Can you work these out from the model? Positions are in its coordinate system, mm. A direction names the side the tool comes from. Give positions to 0.01 mm unless a question says otherwise; leave off trailing zeros. Loops run counter-clockwise (first coordinate to the right, second up) from the corner with the lowest first, then second, coordinate; pieces in that order, holes last. Notation, with made-up numbers: (20.25, 67) -> (44.25, 67) arc R31 cw to (44.25, 101) -> close; hole circle Ø10 at (82, 59.5). An arc over 180 degrees is marked (long way). Use CSV: the item, a comma, the result in double quotes.
from build123d import *

# Parameters (mm, degrees)
SKETCH1_W           = 60
SKETCH1_H           = 60
BOSS_EXTRUDE1_DEPTH = 6
CUT_EXTRUDE2_DEPTH  = 3
SKETCH12_R          = 1.15
CUT_EXTRUDE9_DEPTH  = 43.848570571
SKETCH5_W           = 20
SKETCH5_H           = 60
BOSS_EXTRUDE2_DEPTH = 7
SKETCH6_R           = 1.15
CUT_EXTRUDE4_DEPTH  = 45.373415465
SKETCH8_R           = 2.2
SKETCH8_R_2         = 1.15
CUT_EXTRUDE5_DEPTH  = 9
CUT_EXTRUDE6_DEPTH  = 10
SKETCH10_W          = 6
SKETCH10_H          = 33.5
CUT_EXTRUDE7_DEPTH  = 3
CUT_EXTRUDE8_DEPTH  = 66.711490624


with BuildPart() as part:
    # Sketch1 → Boss-Extrude1 (new body)
    with BuildSketch(Plane.XY):
        Rectangle(SKETCH1_W, SKETCH1_H)
    extrude(amount=BOSS_EXTRUDE1_DEPTH)

    # Sketch3 → Cut-Extrude2 (cut)
    with BuildSketch(Plane(origin=(0, 0, 0), x_dir=(-1, 0, 0), z_dir=(0, 0, -1))):
        Polygon((2.1, 6.287564435), (2.1, 8.712435565), (0, 9.924871131), (-2.1, 8.712435565), (-2.1, 6.287564435), (0, 5.075128869), align=None)
        Polygon((2.1, -8.712435565), (2.1, -6.287564435), (0, -5.075128869), (-2.1, -6.287564435), (-2.1, -8.712435565), (0, -9.924871131), align=None)
        Polygon((2.1, -23.712435565), (2.1, -21.287564435), (0, -20.075128869), (-2.1, -21.287564435), (-2.1, -23.712435565), (0, -24.924871131), align=None)
        Polygon((0, 20.075128869), (2.1, 21.287564435), (2.1, 23.712435565), (0, 24.924871131), (-2.1, 23.712435565), (-2.1, 21.287564435), align=None)
    extrude(amount=-CUT_EXTRUDE2_DEPTH, mode=Mode.SUBTRACT)

    # Sketch12 → Cut-Extrude9 (cut, through all)
    with BuildSketch(Plane(origin=(0, 0, 0), x_dir=(-1, 0, 0), z_dir=(0, 0, -1))):
        with Locations((0, 22.5)):
            Circle(SKETCH12_R)
        with Locations((0, 7.5)):
            Circle(SKETCH12_R)
        with Locations((0, -7.5)):
            Circle(SKETCH12_R)
        with Locations((0, -22.5)):
            Circle(SKETCH12_R)
    extrude(amount=-CUT_EXTRUDE9_DEPTH, mode=Mode.SUBTRACT)

    # Sketch5 → Boss-Extrude2 (add)
    with BuildSketch(Plane.XY.offset(6)):
        with Locations((-20, 0)):
            Rectangle(SKETCH5_W, SKETCH5_H)
        with Locations((20, 0)):
            Rectangle(SKETCH5_W, SKETCH5_H)
    extrude(amount=BOSS_EXTRUDE2_DEPTH)

    # Sketch6 → Cut-Extrude4 (cut, through all)
    with BuildSketch(Plane.XY.offset(13)):
        with Locations((-25, 25)):
            Circle(SKETCH6_R)
        with Locations((25, 25)):
            Circle(SKETCH6_R)
        with Locations((25, -25)):
            Circle(SKETCH6_R)
        with Locations((-25, -25)):
            Circle(SKETCH6_R)
    extrude(amount=-CUT_EXTRUDE4_DEPTH, mode=Mode.SUBTRACT)

    # Sketch8 → Cut-Extrude5 (cut)
    # profile 1 of 4: a face of its own
    with BuildSketch(Plane.XY.offset(13)):
        with Locations((-25, 25)):
            Circle(SKETCH8_R)
        with Locations((-25, 25)):
            Circle(SKETCH8_R_2, mode=Mode.SUBTRACT)
    # profile 2 of 4: a face of its own
    with BuildSketch(Plane.XY.offset(13)):
        with Locations((25, 25)):
            Circle(SKETCH8_R)
    # profile 3 of 4: a face of its own
    with BuildSketch(Plane.XY.offset(13)):
        with Locations((25, -25)):
            Circle(SKETCH8_R)
    # profile 4 of 4: a face of its own
    with BuildSketch(Plane.XY.offset(13)):
        with Locations((-25, -25)):
            Circle(SKETCH8_R)
        with Locations((-25, -25)):
            Circle(SKETCH8_R_2, mode=Mode.SUBTRACT)
    extrude(amount=-CUT_EXTRUDE5_DEPTH, mode=Mode.SUBTRACT)

    # Sketch9 → Cut-Extrude6 (cut)
    with BuildSketch(Plane.XY.offset(13)):
        Polygon((-25, -16.55), (-15.5, -27), (-10, -27), (-10, 6.5), (-23.375, 6.5), (-25, 4.9), (-25, 3.3), (-27, 3.3), (-27, -3.3), (-25, -3.3), align=None)
    extrude(amount=-CUT_EXTRUDE6_DEPTH, mode=Mode.SUBTRACT)

    # Sketch10 → Cut-Extrude7 (cut)
    with BuildSketch(Plane.XY.offset(6)):
        with Locations((-7, -10.25)):
            Rectangle(SKETCH10_W, SKETCH10_H)
    extrude(amount=-CUT_EXTRUDE7_DEPTH, mode=Mode.SUBTRACT)

    # Sketch11 → Cut-Extrude8 (cut, through all)
    with BuildSketch(Plane(origin=(-27, 0, 0), x_dir=(0, 0, -1), z_dir=(1, 0, 0))):
        with BuildLine():
            Line((-3, -0.899652711), (-3, 0.899652711))
            ThreePointArc((-3, 0.899652711), (-9.475, 0), (-3, -0.899652711))
        make_face()
    extrude(amount=-CUT_EXTRUDE8_DEPTH, mode=Mode.SUBTRACT)


solid = part.part
(1) If we section it at B-B, the plane z = 7.5: Write out the boundary of the cut face in (x, y) (3 decimals), then the cut area to 3 significant figures.
Answer sheet:
outline,"(-30, -30) -> (-10, -30) -> (-10, -27) -> (-15.5, -27) -> (-25, -16.55) -> (-25, -3.3) -> (-27, -3.3) -> (-27, -3.022) -> (-30, -3.022) -> close; (-30, 3.022) -> (-27, 3.022) -> (-27, 3.3) -> (-25, 3.3) -> (-25, 4.9) -> (-23.375, 6.5) -> (-10, 6.5) -> (-10, 30) -> (-30, 30) -> close; (10, -30) -> (30, -30) -> (30, 30) -> (10, 30) -> close; hole circle Ø4.4 at (-25, -25); hole circle Ø4.4 at (-25, 25); hole circle Ø4.4 at (25, -25); hole circle Ø4.4 at (25, 25)"
area,"1,860 mm2"
(2) If we section it at C-C, the plane y = -14: Write out the boundary of the cut face in (x, z).
Answer sheet:
outline,"(-30, 0) -> (30, 0) -> (30, 13) -> (10, 13) -> (10, 6) -> (-4, 6) -> (-4, 3) -> (-25, 3) -> (-25, 13) -> (-30, 13) -> close"
(3) If we section it at D-D, the plane x = 8: Write out the boundary of the cut face in (y, z).
Answer sheet:
outline,"(-30, 0) -> (30, 0) -> (30, 6) -> (-30, 6) -> close"
(4) Will these pins go through, and if not, where does the flat tip stop? pin 1 Ø2 at (x, y) = (0, -7) entering from -Z; pin 2 Ø3.5 at (x, y) = (25, 25) entering from +Z; pin 3 Ø1 at (x, y) = (-7.5, 8) entering from -Z; pin 4 Ø10 at (x, y) = (-2.5, -7.5) entering from +Z.
Answer sheet:
pin 1,"stops at z = 3"
pin 2,"stops at z = 4"
pin 3,"stops at z = 0"
pin 4,"stops at z = 6"
(5) If I drill on L1, parallel to Y at x = 25, z = 8.5; L2, parallel to Y at x = 0, z = 4.7; L3, parallel to Y at x = -25, z = 2.95, over which ranges is the centre line in solid material (lowest first)? Write a range as from..to.
Answer sheet:
L1,"y = -30..-27.2, -22.8..22.8, 27.2..30"
L2,"y = -30..-23.65, -21.35..-8.65, -6.35..6.35, 8.65..21.35, 23.65..30"
L3,"y = -30..-26.15, -23.85..23.85, 26.15..30"
(6) If we section it at A-A, the plane y = 7.5: Write out the boundary of the cut face in (x, z).
Answer sheet:
outline,"(-30, 0) -> (-2.1, 0) -> (-2.1, 3) -> (-1.15, 3) -> (-1.15, 6) -> (-10, 6) -> (-10, 13) -> (-30, 13) -> close; (1.15, 3) -> (2.1, 3) -> (2.1, 0) -> (30, 0) -> (30, 13) -> (10, 13) -> (10, 6) -> (1.15, 6) -> close"
(7) Which directions (+Z, -Z, +X, -X, +Y, -Y) give clear straight access to the entire face, cutting with the end or side of a thin tool? Please do faces 1 (the face through (2.1, -7, 1)), 2 (the face through (-10, 18, 9)), 3 (the face through (-25.477, -27.148, 8.563)).
Answer sheet:
face 1,"-Z"
face 2,"+Z, +Y, -Y"
face 3,"+Z"
